```python
from build123d import *

# Parameters (mm, degrees)
PAD125_DEPTH            = 4
SKETCH248_R             = 12
PAD126_DEPTH            = 12
POCKET089_DEPTH         = 8
SKETCH249_R             = 3.1
POCKET090_DEPTH         = 12.001
SKETCH250_R             = 2.35
POCKET091_DEPTH         = 12.001
SKETCH251_W             = 10
SKETCH251_H             = 6.070738
POCKET092_DEPTH         = 12.001
BODY142_PLACEMENT_ANGLE = 180


with BuildPart() as part:
    # Sketch247 → Pad125 (new body)
    with BuildSketch(Plane.XY):
        Polygon((-3.45, 2), (-3.45, 18.25), (3.45, 18.25), (3.45, 2), (9.95, 2), (9.95, -2), (3.45, -2), (3.45, -18.25), (-3.45, -18.25), (-3.45, -2), (-9.95, -2), (-9.95, 2), align=None)
    extrude(amount=PAD125_DEPTH)

    # Sketch248 (on Face14 of Pad125) → Pad126 (join)
    with BuildSketch(Plane.XY.offset(4)):
        Circle(SKETCH248_R)
    extrude(amount=PAD126_DEPTH)

    # Pad126 Face4 → Pocket089 (cut)
    with BuildSketch(Plane(origin=(0, 0, 0), x_dir=(0, -1, 0), z_dir=(0, 0, -1))):
        Polygon((-2, 3.45), (-18.25, 3.45), (-18.25, -3.45), (-2, -3.45), (-2, -9.95), (2, -9.95), (2, -3.45), (18.25, -3.45), (18.25, 3.45), (2, 3.45), (2, 9.95), (-2, 9.95), align=None)
    extrude(amount=-POCKET089_DEPTH, mode=Mode.SUBTRACT)

    # Sketch249 (on Face9 of Pocket089) → Pocket090 (cut, through all)
    with BuildSketch(Plane.XY.offset(16)):
        Circle(SKETCH249_R)
    extrude(amount=-POCKET090_DEPTH, mode=Mode.SUBTRACT)

    # Sketch250 → Pocket091 (cut, through all)
    with BuildSketch(Plane.XZ):
        with Locations((0, 12)):
            Circle(SKETCH250_R)
    extrude(amount=-POCKET091_DEPTH, mode=Mode.SUBTRACT)

    # Sketch251 (on Face12 of Pocket091) → Pocket092 (cut, through all)
    with BuildSketch(Plane.XY.offset(16)):
        with Locations((0, 13.944081)):
            Rectangle(SKETCH251_W, SKETCH251_H)
    extrude(amount=-POCKET092_DEPTH, mode=Mode.SUBTRACT)


with BuildPart() as part_1:
    # Body142 placement: moved
    add(part.part.moved(Location((0, -90, 0))).rotate(Axis((0, -90, 0), (-1, 0, 0)), BODY142_PLACEMENT_ANGLE))


solid = part_1.part
```
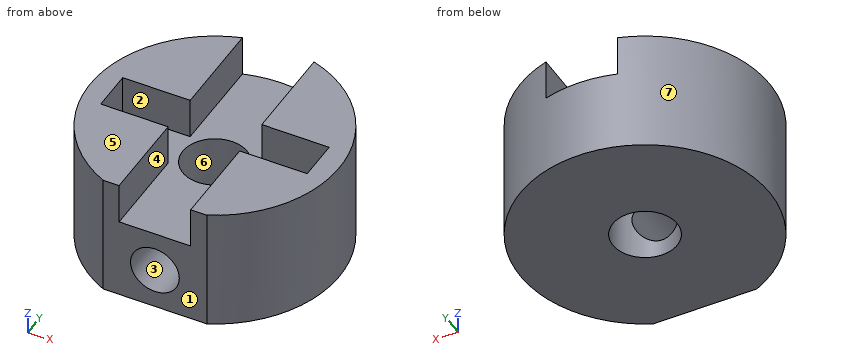
Design review of the part built by this model. Coordinates are the model's own, in mm. Face numbers are marked on the shaded views. A direction names the side the tool comes from. Coordinates: 2 decimals unless noted, no trailing zeros. Write each loop counter-clockwise with the first axis right and the second up, starting at its lowest first coordinate (ties: lowest second). Pieces come first, ordered by that corner, then holes. Notation, with made-up numbers: M 24.25,-0.75 L 65.25,-0.75 A23 ccw 65.25,11.25 Z; hole C 62.5,86 d7. An arc over 180 degrees is marked long. Answer as a JSON object with one key per item and string values.
Item 1: Add section D-D, the plane y = -94.25. Give the boundary of the cut face in (x, z).
Outcome:
{"outline": "M -11.22,-16 L 11.22,-16 L 11.22,-4 L 3.45,-4 L 3.45,-8 L -3.45,-8 L -3.45,-4 L -11.22,-4 Z; hole C 0,-12 d4.7"}
Item 2: Wall thickness on probe 1 along Z at (x, y) = (0, -96); probe 2 along X at (y, z) = (-90, -11.5); probe 3 along Y at (x, z) = (0, -13.75): over which ranges is each line inside the solid? List them lowest first.
Outcome:
{"probe 1": "-16 to -14.35, -9.65 to -8", "probe 2": "-12 to -3.1, 3.1 to 12", "probe 3": "-86.9 to -78"}
Item 3: Add section B-B, the plane y = -90. Give the boundary of the cut face in (x, z), and give its area (3 significant figures).
Outcome:
{"outline": "M -12,-16 L -3.1,-16 L -3.1,-8 L -9.95,-8 L -9.95,-4 L -12,-4 Z; M 3.1,-16 L 12,-16 L 12,-4 L 9.95,-4 L 9.95,-8 L 3.1,-8 Z", "area": "159 mm²"}
Item 4: Draft analysis for pull direction X (two halves, no side actions). For the marked faces 5, 6 and 7, state which applies: pulls with the +X half, pulls with the -X half, needs draft (parallel to the pull), parting line crosses it, or undercut.
Outcome:
{"face 5": "needs draft", "face 6": "undercut", "face 7": "parting line crosses it"}
Item 5: Add section A-A, the plane z = -6.25. Give the boundary of the cut face in (x, y).
Outcome:
{"outline": "M -9.95,-92 L -9.95,-88 L -3.45,-88 L -3.45,-78.51 A12 ccw -5,-100.91 L -3.45,-100.91 L -3.45,-92 Z; M 3.45,-100.91 L 5,-100.91 A12 ccw 3.45,-78.51 L 3.45,-88 L 9.95,-88 L 9.95,-92 L 3.45,-92 Z"}
Item 6: Machinability: for the marked faces 1, 2, 3 and 4, which of the approach directions +Z, -Z, +X, -X, +Y, -Y give a long, thin tool a straight path to every point of the face, cutting with its end or side? Answer none if there is none.
Outcome:
{"face 1": "+Z, -Z, +X, -X, -Y", "face 2": "+Z", "face 3": "-Y", "face 4": "+Z, +Y, -Y"}
Item 7: Add section C-C, the plane x = 0. Give the boundary of the cut face in (y, z), and give its area (3 significant figures).
Outcome:
{"outline": "M -100.91,-16 L -93.1,-16 L -93.1,-14.35 L -100.91,-14.35 Z; M -100.91,-9.65 L -93.1,-9.65 L -93.1,-8 L -100.91,-8 Z; M -86.9,-16 L -78,-16 L -78,-8 L -86.9,-8 Z", "area": "97.0 mm²"}
Item 8: Insertion check: pin 1 Ø2 at (y, z) = (-81.5, -6.5) entering from +X; pin 2 Ø2 at (y, z) = (-85.5, -5.5) entering from -X; pin 3 Ø4 at (y, z) = (-94.5, -10.5) entering from -X. Each pin has a flat end and moves straight along its axis. Give the tip position at first contact, or say it passes through.
Outcome:
{"pin 1": "x = 9.37", "pin 2": "x = -11.48", "pin 3": "x = -11.74"}
